Here's how the part is built. I have some questions about the finished solid (model axes, mm). A direction names the side the tool comes from. Give positions to 0.01 mm unless a question says otherwise; leave off trailing zeros. Order: outer loops, then holes, each group sorted by start corner. A loop starts at its lowest first (then second) coordinate and runs counter-clockwise, first axis right, second up.
from build123d import *

# Parameters (mm, degrees)
SKETCH_1_R      = 2
SKETCH_1_R_2    = 1.75
SKETCH_1_R_3    = 25
SKETCH_1_R_4    = 1.6
SKETCH_1_R_5    = 2.6
EXTRUDE_1_DEPTH = 5
FILLET_1_R      = 20


with BuildPart() as part:
    # 草图1 → 凸台-拉伸1 (new body)
    with BuildSketch(Plane.XY):
        Polygon((0, 108.239220029), (-76.536686473, 76.536686473), (-108.239220029, 0), (-76.536686473, -76.536686473), (0, -108.239220029), (76.536686473, -76.536686473), (108.239220029, 0), (76.536686473, 76.536686473), align=None)
        with Locations((-35.206875778, -84.996916991)):
            Circle(SKETCH_1_R, mode=Mode.SUBTRACT)
        with Locations((84.996916991, -35.206875778)):
            Circle(SKETCH_1_R, mode=Mode.SUBTRACT)
        with Locations((35.206875778, 84.996916991)):
            Circle(SKETCH_1_R, mode=Mode.SUBTRACT)
        with Locations((-84.996916991, 35.206875778)):
            Circle(SKETCH_1_R, mode=Mode.SUBTRACT)
        with Locations((-58.002770081, 35.506036994)):
            Circle(SKETCH_1_R_2, mode=Mode.SUBTRACT)
        with Locations((-15.90759252, -66.120711583)):
            Circle(SKETCH_1_R_2, mode=Mode.SUBTRACT)
        with Locations((58.002770081, -35.506036994)):
            Circle(SKETCH_1_R_2, mode=Mode.SUBTRACT)
        with Locations((15.90759252, 66.120711583)):
            Circle(SKETCH_1_R_2, mode=Mode.SUBTRACT)
        with Locations((89.588318422, -20.926853617)):
            Circle(SKETCH_1_R, mode=Mode.SUBTRACT)
        with Locations((-20.926853617, -89.588318422)):
            Circle(SKETCH_1_R, mode=Mode.SUBTRACT)
        with Locations((-89.588318422, 20.926853617)):
            Circle(SKETCH_1_R, mode=Mode.SUBTRACT)
        with Locations((20.926853617, 89.588318422)):
            Circle(SKETCH_1_R, mode=Mode.SUBTRACT)
        with Locations((-48.55098737, -78.146027573)):
            Circle(SKETCH_1_R, mode=Mode.SUBTRACT)
        with Locations((-78.146027573, 48.55098737)):
            Circle(SKETCH_1_R, mode=Mode.SUBTRACT)
        with Locations((48.55098737, 78.146027573)):
            Circle(SKETCH_1_R, mode=Mode.SUBTRACT)
        Circle(SKETCH_1_R_3, mode=Mode.SUBTRACT)
        with Locations((-34.441508913, 83.149157926)):
            Circle(SKETCH_1_R_4, mode=Mode.SUBTRACT)
        with Locations((-28.701257427, 69.290964938)):
            Circle(SKETCH_1_R_5, mode=Mode.SUBTRACT)
        with Locations((30.614674589, -73.910362601)):
            Circle(SKETCH_1_R_4, mode=Mode.SUBTRACT)
        with Locations((34.441508913, -83.149157926)):
            Circle(SKETCH_1_R_5, mode=Mode.SUBTRACT)
        with BuildLine():
            Line((-62.097714236, -6.870411885), (-48.767829666, -39.051599999))
            ThreePointArc((-48.767829666, -39.051599999), (-55.532780918, -55.38363706), (-71.864817978, -48.618685808))
            Line((-71.864817978, -48.618685808), (-85.194702548, -16.437497694))
            ThreePointArc((-85.194702548, -16.437497694), (-78.429751297, -0.105460633), (-62.097714236, -6.870411885))
        make_face(mode=Mode.SUBTRACT)
        with BuildLine():
            Line((48.767829666, 39.051599999), (62.097714236, 6.870411885))
            ThreePointArc((62.097714236, 6.870411885), (78.429751297, 0.105460633), (85.194702548, 16.437497694))
            Line((85.194702548, 16.437497694), (71.864817978, 48.618685808))
            ThreePointArc((71.864817978, 48.618685808), (55.532780918, 55.38363706), (48.767829666, 39.051599999))
        make_face(mode=Mode.SUBTRACT)
    extrude(amount=EXTRUDE_1_DEPTH)

    # 圆角1
    fillet_1_edges = [part.edges().sort_by_distance(p)[0] for p in [
        (76.536686473, 76.536686473, 2.5),
        (108.239220029, 0, 2.5),
        (76.536686473, -76.536686473, 2.5),
        (0, -108.239220029, 2.5),
        (-76.536686473, -76.536686473, 2.5),
        (-108.239220029, 0, 2.5),
        (-76.536686473, 76.536686473, 2.5),
        (0, 108.239220029, 2.5),
    ]]
    fillet(fillet_1_edges, radius=FILLET_1_R)


solid = part.part
Q1. I'm going to push flat-ended pins straight in: P1, Ø5.5, axis at x = 15.91, y = 66.12, coming from the +Z side; P2, Ø2, axis at x = 26, z = 1, coming from the -Y side; P3, Ø1.5, axis at y = -72, z = 2, coming from the -X side; P4, Ø1.5, axis at y = -34.5, z = 3, coming from the -X side. Where does each tip first touch, or does it pass through?
Filled sheet:
P1: stops at z = 5
P2: stops at y = -97.88
P3: stops at x = -78.54
P4: stops at x = -94.26
Q2. If we section it at A-A on x = 0: List the corners of the cut face in (y, z) for me, plus the area to 3 significant figures.
Filled sheet:
outline: (-106.59, 0) - (-25, 0) - (-25, 5) - (-106.59, 5) - close; (25, 0) - (106.59, 0) - (106.59, 5) - (25, 5) - close
area: 816 mm2
Q3. If we section it at B-B on x = 75: List the corners of the cut face in (y, z) for me.
Filled sheet:
outline: (-75.73, 0) - (-0.77, 0) - (-0.77, 5) - (-75.73, 5) - close; (41.05, 0) - (75.73, 0) - (75.73, 5) - (41.05, 5) - close
Q4. I need wall thicknesses on L1, parallel to X at y = 13, z = 4.7; L2, parallel to X at y = -13.5, z = 1.3; L3, parallel to Y at x = 1, z = 2.9. Which ranges of each line are inside material? Lowest first, please.
Filled sheet:
L1: x = -102.85 to -21.35, 21.35 to 59.56, 86.07 to 102.85
L2: x = -102.65 to -86.01, -59.35 to -21.04, 21.04 to 102.65
L3: y = -106.57 to -24.98, 24.98 to 106.57
Q5. For faces 1 (the face through (38.7, 92.21, 2.46)), 2 (the face through (78.623, 32.303, 2.465)), which set-ups out of +Z, -Z, +X, -X, +Y, -Y let a thin tool reach every point of the face, with its end or its side?
Filled sheet:
face 1: +Z, -Z, +X, +Y
face 2: +Z, -Z
Q6. Thinking about a two-plate mould opening in X: for faces 3 (the face through (-31.3, 69.4, 2.5)), 4 (the face through (-0.11, 106.59, 2.54)), 5 (the face through (-1.5, 25.2, 0)), which applies, released by +X, released by -X, zero draft, split by the parting line, or undercut?
Filled sheet:
face 3: undercut
face 4: split by the parting line
face 5: zero draft
Q7. If we section it at C-C on z = 0.95: Give the number of separate pieces and of enclosed holes in the cut face, plus the area to 3 significant figures.
Filled sheet:
separate pieces: 1
enclosed holes: 22
area: 28,100 mm2
